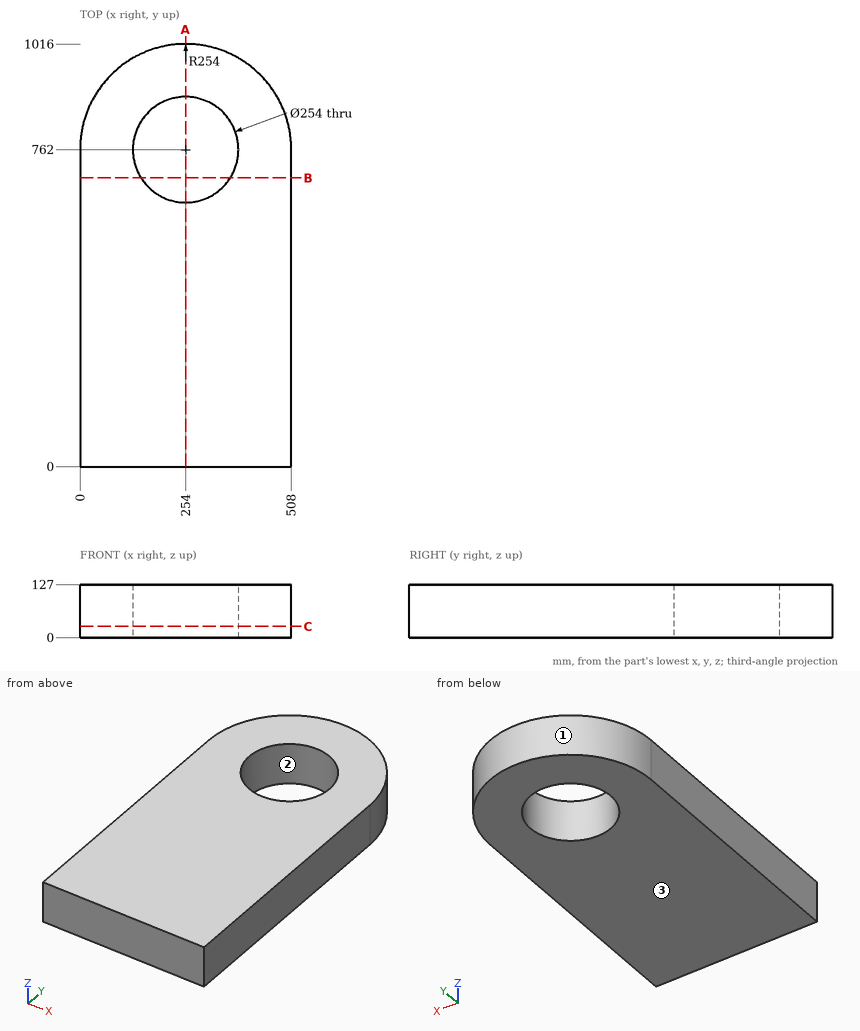
Print and shaded views of the part. All mm, measured from the part's lowest x, y and z. Coordinates: 2 decimals unless noted, no trailing zeros. Order: outer loops, then holes, each group sorted by start corner. A loop starts at its lowest first (then second) coordinate and runs counter-clockwise, first axis right, second up. Notation, with made-up numbers: M 82,-5.75 L 130,-5.75 A18 ccw 130,22.25 Z; hole C 46.5,82 d9. An arc over 180 degrees is marked long. Answer as CSV lines item,"result".
1) Cut at A-A (x = 254). List the corners of the cut face in (y, z), then the cut area to 3 significant figures.
Verdict:
outline,"M 0,0 L 635,0 L 635,127 L 0,127 Z; M 889,0 L 1016,0 L 1016,127 L 889,127 Z"
area,"96,800 mm2"
2) Cut at B-B (y = 694). List the corners of the cut face in (x, z).
Verdict:
outline,"M 0,0 L 146.74,0 L 146.74,127 L 0,127 Z; M 361.26,0 L 508,0 L 508,127 L 361.26,127 Z"
3) Mould opens along Y. For the marked faces 1, 2 and 3 say: released by +Y, released by -Y, zero draft, split by the parting line, or undercut.
Verdict:
face 1,"released by +Y"
face 2,"undercut"
face 3,"zero draft"
4) Cut at C-C (z = 27). List the corners of the cut face in (x, y).
Verdict:
outline,"M 0,0 L 508,0 L 508,762 A254 ccw 0,762 Z; hole C 254,762 d254"
5) Drill centre lines: L1, parallel to X at y = 764.5, z = 29.5; L2, parallel to Y at x = 254, z = 86.5; L3, parallel to Y at x = 365.5, z = 87.5. Where is each one in solid material? Low to high. Write a range as from..to.
Verdict:
L1,"0.01..127.02, 380.98..507.99"
L2,"0..635, 889..1016"
L3,"0..701.2, 822.8..990.22"
6) Flat gauge pin, fed straight in: P1, Ø4, axis at y = 296, z = 80.5, coming from the -X side. Where does the tip first touch, or does it go through?
Verdict:
P1,"x = 0"
